```python
from build123d import *

# Parameters (mm, degrees)
SKETCH2_W           = 1
SKETCH2_H           = 100
BOSS_EXTRUDE1_DEPTH = 150


with BuildPart() as part:
    # Sketch1 → Revolve1 (revolve)
    with BuildSketch(Plane.XY):
        Polygon((0, 0), (-30, 0), (-30, 100), (-5, 100), (-5, 260), (0, 260), align=None)
    revolve(axis=Axis((0, 260, 0), (0, -1, 0)))

    # Sketch2 → Boss-Extrude1 (add)
    with BuildSketch(Plane.XY):
        with Locations((0, 210)):
            Rectangle(SKETCH2_W, SKETCH2_H)
    extrude(amount=BOSS_EXTRUDE1_DEPTH)


solid = part.part
```
The listing builds one solid part. Answer for the finished solid, in the listing's coordinates (mm). A direction names the side the tool comes from. Give positions to 0.01 mm unless a question says otherwise; leave off trailing zeros. Write each loop counter-clockwise with the first axis right and the second up, starting at its lowest first coordinate (ties: lowest second). Pieces come first, ordered by that corner, then holes. Notation, with made-up numbers: M 2.5,11.5 L 12.5,11.5 A24 ccw 12.5,30.5 Z; hole C 35.25,35 d3. An arc over 180 degrees is marked long. Write each question's results on one line, items separated by ' | '.
Q1. Flat-ended cylindrical pins translate along their axes: P1, Ø5, axis at y = 92, z = 17.5, coming from the -X side; P2, Ø1, axis at x = -17.5, y = 51, coming from the -Z side; P3, Ø4, axis at x = -2, y = 162, coming from the -Z side. Find the tip coordinate at first contact, or state that the pin passes through.
Output values:
P1: x = -25.98 | P2: z = -24.72 | P3: z = -5
Q2. A tool of negligible diameter and unlimited length cuts with its end or side. For faces 1 (the flat face through (-0.5, 209, 76)), 2 (the flat face through (0, 260, 49)), 3 (the flat face through (0.5, 209, 76)), from which of +Z, -Z, +X, -X, +Y, -Y can it reach the whole face along a straight path? Write none if from no direction.
Output values:
face 1: +Z, -X, +Y | face 2: +Z, -Z, +X, -X, +Y | face 3: +Z, +X, +Y
Q3. Section D-D, the plane x = -8.5 is taken. Write down the section's boundary in (y, z), then the cut area to 3 significant figures.
Output values:
outline: M 0,-28.77 L 100,-28.77 L 100,28.77 L 0,28.77 Z | area: 5,750 mm2
Q4. Section A-A, the plane z = 0 is taken. Write down the section's boundary in (x, y).
Output values:
outline: M -30,0 L 30,0 L 30,100 L 5,100 L 5,260 L -5,260 L -5,100 L -30,100 Z
Q5. Section C-C, the plane y = 25 is taken. Write down the section's boundary in (x, z).
Output values:
outline: C 0,0 d60
Q6. Consider L1, parallel to X at y = 243.5, z = 30; L2, parallel to Y at x = 6, z = -13.5; L3, parallel to Z at x = 1.5, y = 38. Determine where each line is inside the solid, lowest interval first. Write a range as from..to.
Output values:
L1: -0.5..0.5 | L2: 0..100 | L3: -29.96..29.96
Q7. Section B-B, the plane z = 25.5 is taken. Write down the section's boundary in (x, y), then the cut area to 3 significant figures.
Output values:
outline: M -15.8,0 L 15.8,0 L 15.8,100 L -15.8,100 Z; M -0.5,160 L 0.5,160 L 0.5,260 L -0.5,260 Z | area: 3,260 mm2
